```python
from build123d import *

# Parameters (mm, degrees)
SKETCH_1_W               = 130
SKETCH_1_H               = 20
EXTRUDE_1_DEPTH          = 2
SKETCH_2_W               = 10
SKETCH_2_H               = 6
EXTRUDE_2_DEPTH          = 4
SKETCH_3_R               = 2.5
CUT_EXTRUDE_1_DEPTH      = 4
SKETCH_4_W               = 130
SKETCH_4_H               = 74
SKETCH_4_W_2             = 86
SKETCH_4_H_2             = 56
SKETCH_4_W_3             = 15
SKETCH_4_H_3             = 15
EXTRUDE_3_DEPTH          = 2
EXTRUDE_4_DEPTH          = 2
EXTRUDE_5_DEPTH          = 2
EXTRUDE_6_DEPTH          = 130
SKETCH_9_W               = 10
SKETCH_9_H               = 18
SKETCH_9_W_2             = 12
SKETCH_9_H_2             = 15
EXTRUDE_7_DEPTH          = 4
SKETCH_10_R              = 2.25
CUT_EXTRUDE_2_DEPTH      = 5
CUT_EXTRUDE_3_DEPTH      = 118
CUT_EXTRUDE_3_DEPTH_BACK = 9
FILLET_1_R               = 2
FILLET_2_R               = 2


with BuildPart() as part:
    # Эскиз1 → Бобышка-Вытянуть1 (new body)
    with BuildSketch(Plane(origin=(0, 0, 0), x_dir=(1, 0, 0), z_dir=(0, 1, 0))):
        with Locations((65, 10)):
            Rectangle(SKETCH_1_W, SKETCH_1_H)
    extrude(amount=EXTRUDE_1_DEPTH)

    # Эскиз2 → Бобышка-Вытянуть2 (add)
    with BuildSketch(Plane(origin=(0, 2, 0), x_dir=(1, 0, 0), z_dir=(0, 1, 0))):
        with Locations((5, 10)):
            Rectangle(SKETCH_2_W, SKETCH_2_H)
        with Locations((125, 10)):
            Rectangle(SKETCH_2_W, SKETCH_2_H)
    extrude(amount=EXTRUDE_2_DEPTH)

    # Эскиз3 → Вырез-Вытянуть1 (cut)
    with BuildSketch(Plane(origin=(0, 2, 0), x_dir=(1, 0, 0), z_dir=(0, 1, 0))):
        with Locations(Location((20, 10, 0), (0, 0, 270))):
            Circle(SKETCH_3_R)
        with Locations(Location((110, 10, 0), (0, 0, 270))):
            Circle(SKETCH_3_R)
    extrude(amount=-CUT_EXTRUDE_1_DEPTH, mode=Mode.SUBTRACT)

    # Эскиз4 → Бобышка-Вытянуть3 (add)
    with BuildSketch(Plane(origin=(0, 0.233955557, 0.64278761), x_dir=(1, 0, 0), z_dir=(0, -0.3420201433256631, -0.9396926207859105))):
        with Locations((65, 35.120614758)):
            Rectangle(SKETCH_4_W, SKETCH_4_H)
        with Locations((58, 36.120614758)):
            Rectangle(SKETCH_4_W_2, SKETCH_4_H_2, mode=Mode.SUBTRACT)
        with Locations((116.5, 36.120614758)):
            Rectangle(SKETCH_4_W_3, SKETCH_4_H_3, mode=Mode.SUBTRACT)
    extrude(amount=EXTRUDE_3_DEPTH)

    # Эскиз5 → Бобышка-Вытянуть4 (add)
    with BuildSketch(Plane(origin=(130, 0, 0), x_dir=(0, 0, -1), z_dir=(1, 0, 0))):
        Polygon((0, 2), (-25.309490606, -67.537253938), (20, -88.375754865), (20, 2), align=None)
    extrude(amount=EXTRUDE_4_DEPTH)

    # Эскиз7 → Бобышка-Вытянуть5 (add)
    with BuildSketch(Plane.ZY):
        Polygon((-20, 2), (-20, -88.375754865), (25.309490606, -67.537253938), (0, 2), align=None)
    extrude(amount=EXTRUDE_5_DEPTH)

    # Эскиз8 → Бобышка-Вытянуть6 (add)
    with BuildSketch(Plane.ZY.offset(-130)):
        Polygon((-20, -86.174372086), (22.799977809, -66.490032993), (25.309490606, -67.537253938), (-20, -88.375754865), align=None)
    extrude(amount=EXTRUDE_6_DEPTH)

    # Эскиз9 → Бобышка-Вытянуть7 (add)
    with BuildSketch(Plane(origin=(0, -0.45008473, -1.236597632), x_dir=(-1, 0, 0), z_dir=(0, -0.34202014332566316, -0.9396926207859104))):
        with Locations((-125, -7.021029835)):
            Rectangle(SKETCH_9_W, SKETCH_9_H)
        with Locations((-6, -7.021029835)):
            Rectangle(SKETCH_9_W_2, SKETCH_9_H)
        with Locations((-6, -63.778245038)):
            Rectangle(SKETCH_9_W_2, SKETCH_9_H_2)
        with Locations((-125, -63.778245038)):
            Rectangle(SKETCH_9_W, SKETCH_9_H_2)
    extrude(amount=EXTRUDE_7_DEPTH)

    # Эскиз10 → Вырез-Вытянуть2 (cut)
    with BuildSketch(Plane(origin=(0, -1.818165303, -4.995368115), x_dir=(-1, 0, 0), z_dir=(0, -0.3420201433256632, -0.9396926207859104))):
        with Locations(Location((-124.5, -8.620614758, 0), (0, 0, 90))):
            Circle(SKETCH_10_R)
        with Locations(Location((-7.5, -65.620614758, 0), (0, 0, 90))):
            Circle(SKETCH_10_R)
        with Locations(Location((-124.5, -65.620614758, 0), (0, 0, 90))):
            Circle(SKETCH_10_R)
        with Locations(Location((-7.5, -8.620614758, 0), (0, 0, 90))):
            Circle(SKETCH_10_R)
    extrude(amount=-CUT_EXTRUDE_2_DEPTH, mode=Mode.SUBTRACT)

    # Эскиз11 → Вырез-Вытянуть3 (cut, two sides: drawn at the far end of the back side and taken through both)
    with BuildSketch(Plane.ZY.offset(-120).offset(-CUT_EXTRUDE_3_DEPTH_BACK)):
        Polygon((0.737210819, -5.87307888), (2.618321608, -11.041388294), (0.644967104, -11.759630595), (-1.236143684, -6.591321181), align=None)
        Polygon((20.14698757, -59.201002218), (18.173633066, -59.919244519), (20.054743854, -65.087553933), (22.028098358, -64.369311632), align=None)
    extrude(amount=CUT_EXTRUDE_3_DEPTH + CUT_EXTRUDE_3_DEPTH_BACK, mode=Mode.SUBTRACT)

    # Скругление1
    fillet_1_edges = [part.edges().sort_by_distance(p)[0] for p in [
        (66, -66.490032993, 22.799977809),
    ]]
    fillet(fillet_1_edges, radius=FILLET_1_R)

    # Скругление2
    fillet_2_edges = [part.edges().sort_by_distance(p)[0] for p in [
        (65, -67.537253938, 25.309490606),
    ]]
    fillet(fillet_2_edges, radius=FILLET_2_R)


solid = part.part
```
The listing builds one solid part. Answer for the finished solid, in the listing's coordinates (mm). A direction names the side the tool comes from. Give positions to 0.01 mm unless a question says otherwise; leave off trailing zeros. Write each loop counter-clockwise with the first axis right and the second up, starting at its lowest first coordinate (ties: lowest second). Pieces come first, ordered by that corner, then holes. Notation, with made-up numbers: (-21, 86.5) -> (7, 86.5) arc R24 ccw to (7, 101.5) -> close; hole circle Ø7 at (-12.75, 80). An arc over 180 degrees is marked (long way). Write item = value, one per line. Start each with the question number.
1) The part is cut by section B-B, the plane z = -10. Determine the outline of the cut face in (x, y), and give its area (3 significant figures).
2) Straight lines are drawn through the part: line 1 along X through (y, z) = (1.05, -10); line 2 along X through (y, z) = (-52.5, 9); line 3 along X through (y, z) = (-49, 17.5). For each, find the intervals that lie inside material, in ascending order.
3) The part is cut by section A-A, the plane x = 29. Determine the outline of the cut face in (y, z), and give its area (3 significant figures).
4) Which of the six approach directions +Z, -Z, +X, -X, +Y, -Y give full straight-line access (tool end or side, diameter ignored) to faces 1 (the face through (5, 4, -7)), 2 (the face through (126.56, -8.06, -0.7)), 3 (the face through (120, -8, -1))?
5) Each of these flat-tipped pins is pushed along its axis until it touches: pin 1 (2 mm diameter, centred on y = 4.5, z = -11, fed in from -X); pin 2 (8 mm diameter, centred on x = 69, z = -14, fed in from -Y); pin 3 (8 mm diameter, centred on x = 110, z = -10, fed in from +Y); pin 4 (4.5 mm diameter, centred on x = 4, y = 4, fed in from -Z). Where does it stop, or does it pass through?
6) Determine the mould class of faces 4 (the face through (132, -43, -2)), 5 (the face through (101, -34, 12)), 6 (the face through (65.938, -78.201, 2.123)) for opening direction X: +X half, -X half, draft (parallel to the pull), parting line (faces both ways), or undercut.
Solutions:
q1.outline = (-2, -83.78) -> (132, -83.78) -> (132, 2) -> (130, 2) -> (130, 6) -> (120, 6) -> (120, 2) -> (112.5, 2) -> (112.5, 0) -> (130, 0) -> (130, -81.58) -> (0, -81.58) -> (0, 0) -> (17.5, 0) -> (17.5, 2) -> (10, 2) -> (10, 6) -> (0, 6) -> (0, 2) -> (-2, 2) -> close; (22.5, 0) -> (107.5, 0) -> (107.5, 2) -> (22.5, 2) -> close
q1.area = 949 mm²
q2.line_1 = -2 to 17.5, 22.5 to 107.5, 112.5 to 132
q2.line_2 = -2 to 0, 130 to 132
q2.line_3 = -2 to 15, 101 to 132
q3.outline = (-88.38, -20) -> (-86.17, -20) -> (-67.26, 21.13) arc R2 cw to (-64.76, 22.17) -> (-60.7, 20.69) -> (-60.02, 22.57) -> (-65.81, 24.68) arc R2 ccw to (-68.31, 23.64) -> close; (-8.08, 1.54) -> (0, -1.4) -> (0, -20) -> (2, -20) -> (2, 0) -> (-7.4, 3.42) -> close
q3.area = 168 mm²
q4.face_1 = +Z, +X, -X, +Y
q4.face_2 = none
q4.face_3 = -Z
q5.pin_1 = 0
q5.pin_2 = -87.46
q5.pin_3 = 2
q5.pin_4 = -20
q6.face_4 = +X half
q6.face_5 = undercut
q6.face_6 = draft
